The listing builds one solid part. Answer for the finished solid, in the listing's coordinates (mm). Face numbers are marked on the shaded views. A direction names the side the tool comes from. Give positions to 0.01 mm unless a question says otherwise; leave off trailing zeros. Loops run counter-clockwise (first coordinate to the right, second up) from the corner with the lowest first, then second, coordinate; pieces in that order, holes last. Notation, with made-up numbers: (77, -10.75) -> (117, -10.75) arc R18 cw to (117, 18.25) -> close; hole circle Ø10 at (2, 15). An arc over 180 degrees is marked (long way). One line per question, with ' | ' between items. Start each with the question number.
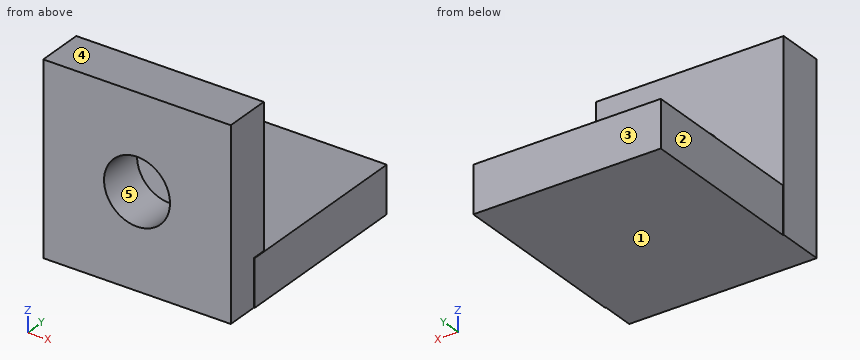
from build123d import *

# Parameters (mm, degrees)
F0_W     = 50.8
F0_H     = 50.8
F1_DEPTH = 12.7
F2_W     = 50.8
F2_H     = 50.8
F2_R     = 8.936433
F3_DEPTH = 12.7
F4_DEPTH = 12.7


with BuildPart() as f1:
    # F0 (on Top) → F1 (new body)
    with BuildSketch(Plane.XY):
        with Locations((-5.648404, 21.607813)):
            Rectangle(F0_W, F0_H)
    extrude(amount=F1_DEPTH)

    # F2 (on Front) → F3 (join)
    with BuildSketch(Plane.XZ):
        with Locations((-5.861539, 25.4)):
            Rectangle(F2_W, F2_H)
        with Locations((-5.861539, 25.4)):
            Circle(F2_R, mode=Mode.SUBTRACT)
    extrude(amount=F3_DEPTH)

    # F2 (on Front) → F4 (join)
    with BuildSketch(Plane.XZ):
        with Locations((-5.861539, 25.4)):
            Rectangle(F2_W, F2_H)
        with Locations((-5.861539, 25.4)):
            Circle(F2_R, mode=Mode.SUBTRACT)
    extrude(amount=F4_DEPTH)


solid = f1.part
1. Straight lines are drawn through the part: L1, parallel to X at y = -3, z = 25; L2, parallel to Y at x = -17, z = 42; L3, parallel to X at y = 8, z = 3. For each, find the intervals that lie inside material, in ascending order.
2. The part is cut by section C-C (x = 6). Write down the section's boundary in (y, z).
3. The part is cut by section D-D (x = -2). Write down the section's boundary in (y, z).
4. For the marked faces 1 and 2, determine the directions among +Z, -Z, +X, -X, +Y, -Y from which every point of the face is accessible in a straight line to the end or side of a thin tool.
5. The part is cut by section A-A (z = 25.4). Write down the section's boundary in (x, y), plus the area to 3 significant figures.
6. Determine the mould class of the marked faces 3, 4 and 5 for opening direction Z: released by +Z, released by -Z, zero draft, split by the parting line, or undercut.
7. Each of these flat-tipped pins is pushed along its axis until it touches: pin 1 Ø10 at (y, z) = (-9, 27) entering from +X; pin 2 Ø4 at (y, z) = (26.5, 11.5) entering from -X; pin 3 Ø1.5 at (x, z) = (-17, 23) entering from +Y. Where does it stop, or does it pass through?
8. The part is cut by section B-B (y = -9). Write down the section's boundary in (x, z), plus the area to 3 significant figures.
Check sheet entries:
1) L1: x = -31.26 to -14.79, 3.07 to 19.54 | L2: y = -12.7 to 0 | L3: x = -31.05 to 19.75
2) outline: (-12.7, 0) -> (47.01, 0) -> (47.01, 12.7) -> (0, 12.7) -> (0, 50.8) -> (-12.7, 50.8) -> close
3) outline: (-12.7, 0) -> (47.01, 0) -> (47.01, 12.7) -> (0, 12.7) -> (0, 17.34) -> (-12.7, 17.34) -> close; (-12.7, 33.46) -> (0, 33.46) -> (0, 50.8) -> (-12.7, 50.8) -> close
4) face 1: -Z, +X, -X, +Y, -Y | face 2: +Z, -Z, -X, +Y
5) outline: (-31.26, -12.7) -> (-14.8, -12.7) -> (-14.8, 0) -> (-31.26, 0) -> close; (3.07, -12.7) -> (19.54, -12.7) -> (19.54, 0) -> (3.07, 0) -> close | area: 418 mm^2
6) face 3: zero draft | face 4: released by +Z | face 5: undercut
7) pin 1: stops at x = 19.54 | pin 2: stops at x = -31.05 | pin 3: stops at y = 0
8) outline: (-31.26, 0) -> (19.54, 0) -> (19.54, 50.8) -> (-31.26, 50.8) -> close; hole circle Ø17.87 at (-5.86, 25.4) | area: 2,330 mm^2
